from build123d import *

# Parameters (mm, degrees)
F0_R     = 14.0159979079
F0_R_2   = 1.6
F1_DEPTH = 3.5
F2_R     = 2


# Not quite as in the source:
# - a feature names something its author has since deleted; it is built from what else it names


with BuildPart() as f1:
    # F0 (on Top) → F1 (new body)
    with BuildSketch(Plane.XY):
        with Locations((4.1739126741, 0)):
            Circle(F0_R)
        with Locations((-0.8260871004, -8.6602539076)):
            Circle(F0_R_2, mode=Mode.SUBTRACT)
        with Locations((-5.8260870252, 0)):
            Circle(F0_R_2, mode=Mode.SUBTRACT)
        with Locations((4.1739126741, 0)):
            Circle(F0_R_2, mode=Mode.SUBTRACT)
        with Locations((9.1739127493, -8.6602539076)):
            Circle(F0_R_2, mode=Mode.SUBTRACT)
        with Locations((14.1739126741, 0)):
            Circle(F0_R_2, mode=Mode.SUBTRACT)
        with Locations((-0.8260871004, 8.6602539076)):
            Circle(F0_R_2, mode=Mode.SUBTRACT)
        with Locations((9.1739127493, 8.6602539076)):
            Circle(F0_R_2, mode=Mode.SUBTRACT)
    extrude(amount=F1_DEPTH)

    # F2
    f2_edges = [f1.edges().sort_by_distance(p)[0] for p in [
        (-9.842085, 0, 3.5),
    ]]
    fillet(f2_edges, radius=F2_R)


solid = f1.part
The listing builds one solid part. Answer for the finished solid, in the listing's coordinates (mm). Coordinates: 2 decimals unless noted, no trailing zeros. Order: outer loops, then holes, each group sorted by start corner. A loop starts at its lowest first (then second) coordinate and runs counter-clockwise, first axis right, second up.
Q1. Given P1, Ø1.5, axis at x = 15, z = 1.5, coming from the -Y side; P2, Ø1, axis at x = 6, z = 1, coming from the +Y side, each flat-ended and moving along its own axis, determine where each tip first touches the part or whether it passes through.
Q2. A cutting plane is placed at C-C, the plane x = 0. State how many separate pieces and enclosed holes the cut face has, and give its area (3 significant figures).
Q3. A cutting plane is placed at A-A, the plane y = 0. Write down the section's boundary in (x, z), and give its area (3 significant figures).
Q4. A cutting plane is placed at D-D, the plane z = 2.75. Write down the section's boundary in (x, y), and give its area (3 significant figures).
Q5. A cutting plane is placed at B-B, the plane z = 0.6. Write down the section's boundary in (x, y).
Q6. For a pull along Y with two mould halves and no side action, classify faces 1 (the face through (9.91, -10.08, 1.73)), 2 (the face through (7, 0, 3.5)), 3 (the face through (17.543, 4.21, 0.74)), 4 (the face through (-7.425, 0.07, 1.726)) as pulls with the +Y half, pulls with the -Y half, needs draft (parallel to the pull), parting line crosses it, or undercut.
Q7. Consider line 1 (X direction, y = -7.5, z = 3.15); line 2 (Y direction, x = -0.5, z = 1.25); line 3 (X direction, y = 7.75, z = 2.75). Determine where each line is inside the solid, lowest interval first.
Answers follow:
1. P1: stops at y = -9.74
1. P2: stops at y = 13.95
2. separate pieces: 3
2. enclosed holes: 0
2. area: 72.7 mm2
3. outline: (-9.84, 0) - (-7.43, 0) - (-7.43, 3.5) - (-7.84, 3.5) arc R2 ccw to (-9.84, 1.5) - close; (-4.23, 0) - (2.57, 0) - (2.57, 3.5) - (-4.23, 3.5) - close; (5.77, 0) - (12.57, 0) - (12.57, 3.5) - (5.77, 3.5) - close; (15.77, 0) - (18.19, 0) - (18.19, 1.5) arc R2 ccw to (16.19, 3.5) - (15.77, 3.5) - close
3. area: 62.8 mm2
4. outline: circle Ø27.15 at (4.17, 0); hole circle Ø3.2 at (-5.83, 0); hole circle Ø3.2 at (-0.83, -8.66); hole circle Ø3.2 at (-0.83, 8.66); hole circle Ø3.2 at (4.17, 0); hole circle Ø3.2 at (9.17, -8.66); hole circle Ø3.2 at (9.17, 8.66); hole circle Ø3.2 at (14.17, 0)
4. area: 523 mm2
5. outline: circle Ø28.03 at (4.17, 0); hole circle Ø3.2 at (-5.83, 0); hole circle Ø3.2 at (-0.83, -8.66); hole circle Ø3.2 at (-0.83, 8.66); hole circle Ø3.2 at (4.17, 0); hole circle Ø3.2 at (9.17, -8.66); hole circle Ø3.2 at (9.17, 8.66); hole circle Ø3.2 at (14.17, 0)
6. face 1: undercut
6. face 2: needs draft
6. face 3: parting line crosses it
6. face 4: undercut
7. line 1: x = -6.62 to -1.93, 0.28 to 8.07, 10.28 to 14.97
7. line 2: y = -13.21 to -10.23, -7.09 to 7.09, 10.23 to 13.21
7. line 3: x = -6.97 to -2.14, 0.49 to 7.86, 10.49 to 15.32
